from build123d import *

# Parameters (mm, degrees)
PAD_DEPTH       = 200
POCKET_DEPTH    = 65.001
POCKET001_DEPTH = 65.001
SKETCH003_R     = 6
POCKET002_DEPTH = 90.001
FILLET_R        = 10
FILLET001_R     = 10


with BuildPart() as part:
    # Sketch → Pad (new body)
    with BuildSketch(Plane.XY):
        Polygon((60, 0), (60, -10), (-60, -10), (-60, 0), (-5, 0), (-5, 80), (5, 80), (5, 0), align=None)
    extrude(amount=PAD_DEPTH)

    # Sketch001 → Pocket (cut, through all)
    with BuildSketch(Plane.YZ.offset(5)):
        Polygon((20, 0), (80, 0), (80, 100), align=None)
    extrude(amount=-POCKET_DEPTH, mode=Mode.SUBTRACT)

    # Sketch002 → Pocket001 (cut, through all)
    with BuildSketch(Plane(origin=(-5, 0, 0), x_dir=(0, -1, 0), z_dir=(-1, 0, 0))):
        with BuildLine():
            ThreePointArc((-20, 155), (-40, 175), (-60, 155))
            Line((-60, 155), (-60, 115))
            ThreePointArc((-60, 115), (-40, 95), (-20, 115))
            Line((-20, 155), (-20, 115))
        make_face()
    extrude(amount=-POCKET001_DEPTH, mode=Mode.SUBTRACT)

    # Sketch003 → Pocket002 (cut, through all)
    with BuildSketch(Plane.XZ.offset(10)):
        with Locations((-40, 180)):
            Circle(SKETCH003_R)
        with Locations((40, 180)):
            Circle(SKETCH003_R)
        with Locations((-40, 20)):
            Circle(SKETCH003_R)
        with Locations((40, 20)):
            Circle(SKETCH003_R)
    extrude(amount=-POCKET002_DEPTH, mode=Mode.SUBTRACT)

    # Fillet
    fillet_edges = [part.edges().sort_by_distance(p)[0] for p in [
        (5, 0, 100),
        (-5, 0, 100),
    ]]
    fillet(fillet_edges, radius=FILLET_R)

    # Fillet001
    fillet001_edges = [part.edges().sort_by_distance(p)[0] for p in [
        (-60, -5, 200),
        (60, -5, 200),
        (60, -5, 0),
        (-60, -5, 0),
        (0, 20, 0),
        (0, 80, 200),
    ]]
    fillet(fillet001_edges, radius=FILLET001_R)


solid = part.part
Read the model definition and answer for the solid it produces. Units are mm, in the model's axes. A direction names the side the tool comes from. Give positions to 0.01 mm unless a question says otherwise; leave off trailing zeros. Write each loop counter-clockwise with the first axis right and the second up, starting at its lowest first coordinate (ties: lowest second). Pieces come first, ordered by that corner, then holes. Notation, with made-up numbers: (-30.5, 1.5) -> (-18.5, 1.5) arc R28 cw to (-18.5, 22.5) -> close; hole circle Ø2 at (-25.5, 79). An arc over 180 degrees is marked (long way). Answer as a JSON object with one key per item and string values. Group by question number.
1) Find section A-A (z = 20). Write down the section's boundary in (x, y).
2) A tool of negligible diameter and unlimited length cuts with its end or side. For faces 5 (the flat face through (-5, 52.3, 98.6)), 6 (the flat face through (5, 53, 99)), 7 (the cylindrical face through (56.99, -5.07, 2.85)), from which of +Z, -Z, +X, -X, +Y, -Y can it reach the whole face along a straight path? Write none if from no direction.
3) The mould has two halves that part along Y. Classify faces 1 (the cylindrical face through (0.07, 76.99, 197.15)), 2 (the cylindrical face through (0, 40, 95)), 3 (the flat face through (0, 12, 200)), 4 (the flat face through (0, 20, 135)): +Y half, -Y half, draft (parallel to the pull), parting line (faces both ways), or undercut.
4) Find section B-B (x = -40). Write down the section's boundary in (y, z).
5) Find section D-D (z = 142). Write down the section's boundary in (x, y), and give its area (3 significant figures).
6) Each of these flat-tipped pins is pushed along its axis until it touches: P1, Ø15.5, axis at x = -40, z = 180, coming from the +Y side; P2, Ø15.5, axis at x = 40, z = 180, coming from the -Y side; P3, Ø1.5, axis at y = 27, z = 22, coming from the -X side; P4, Ø1.5, axis at y = 11.5, z = 57, coming from the +X side. Where does it stop, or does it pass through?
7) Consider L1, parallel to Z at x = -40, y = -4.25; L2, parallel to Y at x = 31.5, z = 61; L3, parallel to X at y = 35.5, z = 179.5. Determine where each line is inside the solid, lowest interval first. Write a range as from..to.
8) Find section C-C (y = 31.5). Write down the section's boundary in (x, z).
Values follow:
{
 "1": {"outline": "(-60, -10) -> (-46, -10) -> (-46, 0) -> (-60, 0) -> close; (-34, -10) -> (34, -10) -> (34, 0) -> (15, 0) arc R10 cw to (5, 10) -> (5, 32) -> (-5, 32) -> (-5, 10) arc R10 cw to (-15, 0) -> (-34, 0) -> close; (46, -10) -> (60, -10) -> (60, 0) -> (46, 0) -> close"},
 "2": {"face 5": "+Z, -Z, -X, +Y", "face 6": "+Z, -Z, +X, +Y", "face 7": "-Z, +X, +Y, -Y"},
 "3": {"face 1": "+Y half", "face 2": "undercut", "face 3": "draft", "face 4": "undercut"},
 "4": {"outline": "(-10, 0) -> (0, 0) -> (0, 14) -> (-10, 14) -> close; (-10, 26) -> (0, 26) -> (0, 174) -> (-10, 174) -> close; (-10, 186) -> (0, 186) -> (0, 200) -> (-10, 200) -> close"},
 "5": {"outline": "(-60, -10) -> (60, -10) -> (60, 0) -> (15, 0) arc R10 cw to (5, 10) -> (5, 20) -> (-5, 20) -> (-5, 10) arc R10 cw to (-15, 0) -> (-60, 0) -> close; (-5, 60) -> (5, 60) -> (5, 80) -> (-5, 80) -> close", "area": "1,640 mm2"},
 "6": {"P1": "stops at y = 0", "P2": "stops at y = -10", "P3": "stops at x = -5", "P4": "stops at x = 5"},
 "7": {"L1": "z = 0..14, 26..174, 186..200", "L2": "y = -10..0", "L3": "x = -5..5"},
 "8": {"outline": "(-5, 19.17) -> (5, 19.17) -> (5, 96.9) -> (-5, 96.9) -> close; (-5, 173.1) -> (5, 173.1) -> (5, 200) -> (-5, 200) -> close"}
}
